Check sheet for the drawn part. Datum: minimum x, y, z corner. Units: mm. Give positions to 0.01 mm unless a question says otherwise; leave off trailing zeros. Write each loop counter-clockwise with the first axis right and the second up, starting at its lowest first coordinate (ties: lowest second). Pieces come first, ordered by that corner, then holes. Notation, with made-up numbers: M 56.5,29 L 62.5,29 A22 cw 62.5,39 Z; hole C 63,45 d2. An arc over 180 degrees is marked long. Write item = value, one per line.
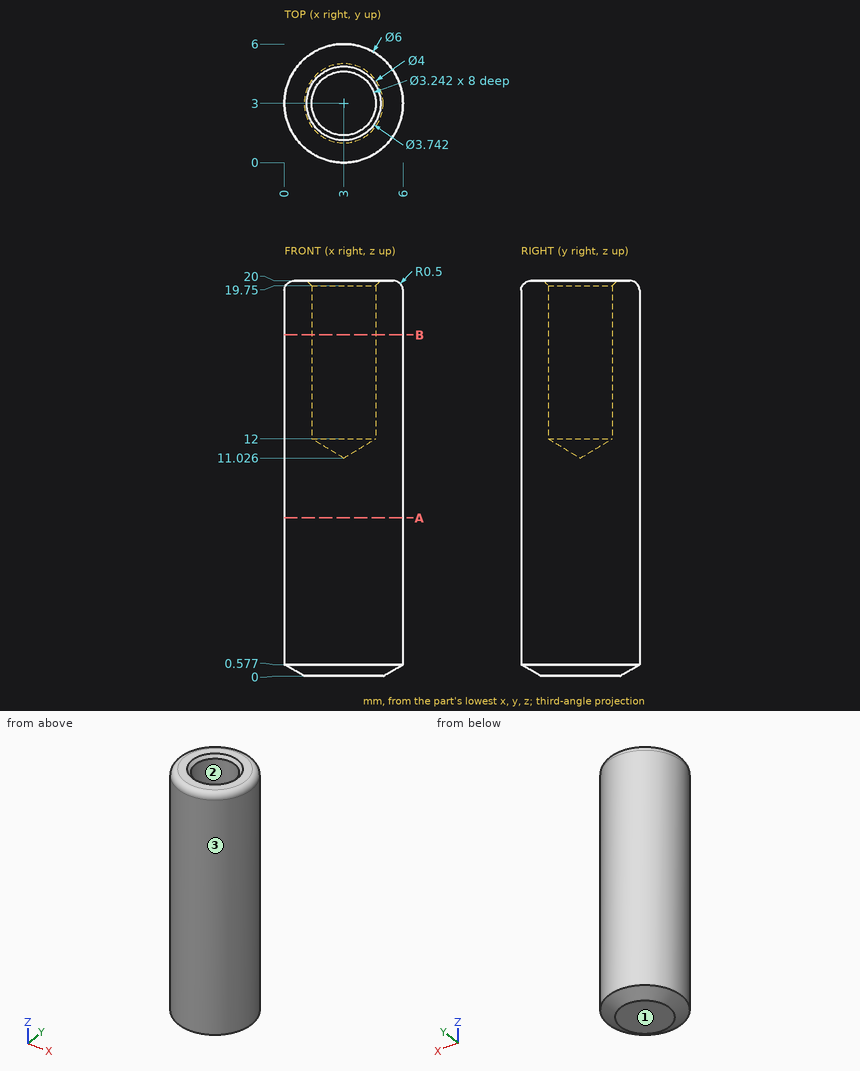
1) Cross-section at A-A on z = 8. Record the boundary of the cut face in (x, y).
From the geometry:
outline = C 3,3 d6
2) Draft check along Y on the marked faces 1, 2 and 3. Enter one of: +Y half, -Y half, draft (parallel to the pull), parting line (faces both ways), or undercut.
From the geometry:
face_1 = draft
face_2 = undercut
face_3 = parting line
3) Depth check by flat-ended pin: P1, Ø1.5, axis at y = 1, z = 9.5, coming from the -X side; P2, Ø1, axis at x = 1, z = 2, coming from the -Y side; P3, Ø3, axis at x = 1, z = 10.5, coming from the +Y side. Enter the tip coordinate at first touch or a pass-through.
From the geometry:
P1 = 0.27
P2 = 0.4
P3 = 5.96
4) Material ranges on probe 1 along X at (y, z) = (3, 18); probe 2 along X at (y, z) = (4.1, 15), recorded low to high. Write a range as from..to.
From the geometry:
probe_1 = 0..1.38, 4.62..6
probe_2 = 0.21..1.81, 4.19..5.79
5) Cross-section at B-B on z = 17.25. Record the boundary of the cut face in (x, y), plus the area to 3 significant figures.
From the geometry:
outline = C 3,3 d6; hole C 3,3 d3.24
area = 20.0 mm^2
